from build123d import *

# Parameters (mm, degrees)
SKETCH1_R           = 20.05
SKETCH1_R_2         = 8
BOSS_EXTRUDE1_DEPTH = 8
SKETCH2_R           = 20.05
SKETCH2_R_2         = 8
SKETCH2_R_3         = 20
BOSS_EXTRUDE2_DEPTH = 7
BOSS_EXTRUDE3_START = -2
SKETCH3_R           = 8
SKETCH3_R_2         = 6
BOSS_EXTRUDE3_DEPTH = 2
SKETCH4_R           = 2.5
SKETCH4_R_2         = 1.5
CUT_EXTRUDE1_DEPTH  = 33.0781078
SKETCH5_R           = 2.5
CUT_EXTRUDE2_DEPTH  = 8
CIRPATTERN1_COUNT   = 3
FILLET1_R           = 2
BOSS_EXTRUDE4_START = -1
SKETCH6_R           = 22
SKETCH6_R_2         = 20.05
BOSS_EXTRUDE4_DEPTH = 1
SKETCH7_R           = 2.5
CUT_EXTRUDE3_DEPTH  = 33.124756808


with BuildPart() as part:
    # Sketch1 → Boss-Extrude1 (new body)
    with BuildSketch(Plane(origin=(0, 0, 0), x_dir=(1, 0, 0), z_dir=(0, 1, 0))):
        with Locations(Location((0, 0, 0), (0, 0, 270))):
            Circle(SKETCH1_R)
        with Locations(Location((0, 0, 0), (0, 0, 270))):
            Circle(SKETCH1_R_2, mode=Mode.SUBTRACT)
    extrude(amount=BOSS_EXTRUDE1_DEPTH)

    # Sketch2 → Boss-Extrude2 (add)
    # profile 1 of 2: a face of its own
    with BuildSketch(Plane(origin=(0, 8, 0), x_dir=(1, 0, 0), z_dir=(0, 1, 0))):
        with Locations(Location((0, 0, 0), (0, 0, 270))):
            Circle(SKETCH2_R)
        with Locations(Location((0, 0, 0), (0, 0, 270))):
            Circle(SKETCH2_R_2, mode=Mode.SUBTRACT)
    # profile 2 of 2: a face of its own
    with BuildSketch(Plane(origin=(0, 8, 0), x_dir=(1, 0, 0), z_dir=(0, 1, 0))):
        with Locations(Location((0, 0, 0), (0, 0, 270))):
            Circle(SKETCH2_R)
        Circle(SKETCH2_R_3, mode=Mode.SUBTRACT)
    extrude(amount=BOSS_EXTRUDE2_DEPTH)

    # Sketch3 → Boss-Extrude3 (add)
    with BuildSketch(Plane(origin=(0, 15, 0), x_dir=(1, 0, 0), z_dir=(0, 1, 0)).offset(BOSS_EXTRUDE3_START)):
        with Locations(Location((0, 0, 0), (0, 0, 270))):
            Circle(SKETCH3_R)
        with Locations(Location((0, 0, 0), (0, 0, 270))):
            Circle(SKETCH3_R_2, mode=Mode.SUBTRACT)
    extrude(amount=BOSS_EXTRUDE3_DEPTH)

    # Sketch4 → Cut-Extrude1 (cut, through all)
    with BuildSketch(Plane(origin=(0, 15, 0), x_dir=(1, 0, 0), z_dir=(0, 1, 0))):
        with Locations(Location((0, 16.5, 0), (0, 0, 270))):
            Circle(SKETCH4_R)
        with Locations(Location((14.289419162, -8.25, 0), (0, 0, 270))):
            Circle(SKETCH4_R)
        with Locations(Location((-14.289419162, -8.25, 0), (0, 0, 270))):
            Circle(SKETCH4_R)
        with Locations(Location((0, -16.5, 0), (0, 0, 270))):
            Circle(SKETCH4_R_2)
        with Locations(Location((-14.289419162, 8.25, 0), (0, 0, 270))):
            Circle(SKETCH4_R_2)
        with Locations(Location((14.289419162, 8.25, 0), (0, 0, 270))):
            Circle(SKETCH4_R_2)
    extrude(amount=-CUT_EXTRUDE1_DEPTH, mode=Mode.SUBTRACT)

    # Sketch5 → Cut-Extrude2 (cut)
    with BuildSketch(Plane.XZ):
        with BuildLine():
            ThreePointArc((-3.332922817, 7.272662889), (-2.919714264, 7.448172166), (-2.497311128, 7.600226124))
            Line((-2.497311128, 7.600226124), (-6.258886015, 19.048066722))
            ThreePointArc((-6.258886015, 19.048066722), (-7.661105353, 18.52862555), (-9.020711712, 17.906123539))
            ThreePointArc((-9.020711712, 17.906123539), (-17.363809346, 10.025), (-20.017513724, -1.140896267))
            ThreePointArc((-20.017513724, -1.140896267), (-19.8768131, -2.629600918), (-19.625552682, -4.103679072))
            Line((-19.625552682, -4.103679072), (-7.830644462, -1.637378184))
            ThreePointArc((-7.830644462, -1.637378184), (-7.91016344, -1.195539359), (-7.964772223, -0.749935616))
            ThreePointArc((-7.964772223, -0.749935616), (-6.92820323, 4), (-3.332922817, 7.272662889))
        make_face()
        with Locations(Location((-14.289419162, 8.25, 0), (0, 0, 90))):
            Circle(SKETCH5_R, mode=Mode.SUBTRACT)
    cut_extrude2 = extrude(amount=-CUT_EXTRUDE2_DEPTH, mode=Mode.SUBTRACT)

    # CirPattern1: Cut-Extrude2 ×3 about axis
    cirpattern1_axis = Axis((0, 0, 0), (0, 1, 0))
    for i in range(1, CIRPATTERN1_COUNT):
        add(cut_extrude2.rotate(cirpattern1_axis, i * 360 / CIRPATTERN1_COUNT), mode=Mode.SUBTRACT)

    # Fillet1
    fillet1_edges = [part.edges().sort_by_distance(p)[0] for p in [
        (-7.830644462, 4, -1.637378184),
        (-19.625552682, 4, -4.103679072),
        (-6.258886015, 4, 19.048066722),
        (-2.497311128, 4, 7.600226124),
        (2.497311128, 4, 7.600226124),
        (6.258886015, 4, 19.048066722),
        (19.625552682, 4, -4.103679072),
        (7.830644462, 4, -1.637378184),
        (5.333333333, 4, -5.96284794),
        (13.366666667, 4, -14.94438765),
        (-13.366666667, 4, -14.94438765),
        (-5.333333333, 4, -5.96284794),
    ]]
    fillet(fillet1_edges, radius=FILLET1_R)

    # Sketch6 → Boss-Extrude4 (add)
    with BuildSketch(Plane(origin=(0, 15, 0), x_dir=(1, 0, 0), z_dir=(0, 1, 0)).offset(BOSS_EXTRUDE4_START)):
        with Locations(Location((0, 0, 0), (0, 0, 270))):
            Circle(SKETCH6_R)
        with Locations(Location((0, 0, 0), (0, 0, 41.828059361))):
            Circle(SKETCH6_R_2, mode=Mode.SUBTRACT)
    extrude(amount=BOSS_EXTRUDE4_DEPTH)

    # Sketch7 → Cut-Extrude3 (cut, through all)
    # profile 1 of 2: a face of its own
    with BuildSketch(Plane.XZ.offset(-8)):
        with BuildLine():
            ThreePointArc((4.109756896, 19.624280834), (5.43201172, 18.666478367), (5.599862615, 17.042418804))
            Line((5.599862615, 17.042418804), (3.058568997, 9.308337966))
            ThreePointArc((3.058568997, 9.308337966), (2.235430366, 8.247362264), (0.926809973, 7.946132599))
            ThreePointArc((0.926809973, 7.946132599), (6.92820323, 4), (7.344957679, -3.170425319))
            ThreePointArc((7.344957679, -3.170425319), (8.260140418, -2.187741646), (9.590541644, -2.005370533))
            Line((9.590541644, -2.005370533), (17.559098934, -3.67158612))
            ThreePointArc((17.559098934, -3.67158612), (18.881650325, -4.62897904), (19.050004181, -6.252986541))
            ThreePointArc((19.050004181, -6.252986541), (17.363809346, 10.025), (4.109756896, 19.624280834))
        make_face()
        with Locations(Location((14.289419162, 8.25, 0), (0, 0, 90))):
            Circle(SKETCH7_R, mode=Mode.SUBTRACT)
    # profile 2 of 2: a face of its own
    with BuildSketch(Plane.XZ.offset(-8)):
        with BuildLine():
            ThreePointArc((5.599862615, 17.042418804), (5.43201172, 18.666478367), (4.109756896, 19.624280834))
            ThreePointArc((4.109756896, 19.624280834), (-17.363809346, -10.025), (19.050004181, -6.252986541))
            ThreePointArc((19.050004181, -6.252986541), (18.881650325, -4.62897904), (17.559098934, -3.67158612))
            Line((17.559098934, -3.67158612), (9.590541644, -2.005370533))
            ThreePointArc((9.590541644, -2.005370533), (8.260140418, -2.187741646), (7.344957679, -3.170425319))
            ThreePointArc((7.344957679, -3.170425319), (-6.92820323, -4), (0.926809973, 7.946132599))
            ThreePointArc((0.926809973, 7.946132599), (2.235430366, 8.247362264), (3.058568997, 9.308337966))
            Line((3.058568997, 9.308337966), (5.599862615, 17.042418804))
        make_face()
    extrude(amount=CUT_EXTRUDE3_DEPTH, mode=Mode.SUBTRACT)


solid = part.part
Build history of the part. All positions in model axes, mm. A direction names the side the tool comes from. Coordinates: 2 decimals unless noted, no trailing zeros. Order: outer loops, then holes, each group sorted by start corner. A loop starts at its lowest first (then second) coordinate and runs counter-clockwise, first axis right, second up. Notation, with made-up numbers: (36, 49) -> (61, 49) arc R16 cw to (61, 58) -> close; hole circle Ø6 at (27.5, 70.5). An arc over 180 degrees is marked (long way). One line per item, written item: value.
(1) Mould opens along Z. For faces 1 (the flat face through (-5, 15, 5)), 2 (the cylindrical face through (6.022, 10.958, 19.124)), 3 (the cylindrical face through (15.777, 11.549, -8.445)) say: pulls with the +Z half, pulls with the -Z half, needs draft (parallel to the pull), parting line crosses it, or undercut.
Checked values:
face 1: needs draft
face 2: parting line crosses it
face 3: undercut
(2) Slice it at B-B, the plane z = 0. List the corners of the cut face in (x, y), plus the area to 3 significant figures.
Checked values:
outline: (-22, 14) -> (-20.05, 14) -> (-20.05, 8) -> (-8, 8) -> (-8, 13) -> (-6, 13) -> (-6, 15) -> (-22, 15) -> close; (6, 13) -> (8, 13) -> (8, 8) -> (20.05, 8) -> (20.05, 14) -> (22, 14) -> (22, 15) -> (6, 15) -> close
area: 181 mm2
(3) Slice it at C-C, the plane y = 9.5. List the corners of the cut face in (x, z), plus the area to 3 significant figures.
Checked values:
outline: circle Ø40.1 at (0, 0); hole circle Ø5 at (-14.29, 8.25); hole circle Ø3 at (-14.29, -8.25); hole circle Ø16 at (0, 0); hole circle Ø5 at (0, -16.5); hole circle Ø3 at (0, 16.5); hole circle Ø5 at (14.29, 8.25); hole circle Ø3 at (14.29, -8.25)
area: 982 mm2
(4) Probe line 1 (X direction, y = 14.5, z = 0); line 2 (X direction, y = 10.5, z = 8.25); line 3 (X direction, y = 10, z = -8.25). List the from-to ranges inside material, lowest first. Write a range as [from, to].
Checked values:
line 1: [-22, -6], [6, 22]
line 2: [-18.27, -16.79], [-11.79, 11.79], [16.79, 18.27]
line 3: [-18.27, -15.79], [-12.79, 12.79], [15.79, 18.27]
(5) Tool access for faces 4 (the flat face through (-10, 14, 18)), 5 (the cylindrical face through (0, 12, 15)): list every direction of +Z, -Z, +X, -X, +Y, -Y with a clear straight run to the whole face (end or side of a thin tool).
Checked values:
face 4: -Y
face 5: +Y, -Y
(6) Slice it at D-D, the plane z = 16.5. List the corners of the cut face in (x, y), plus the area to 3 significant figures.
Checked values:
outline: (-14.55, 14) -> (-11.39, 14) -> (-11.39, 8) -> (-1.5, 8) -> (-1.5, 15) -> (-14.55, 15) -> close; (1.5, 8) -> (11.39, 8) -> (11.39, 14) -> (14.55, 14) -> (14.55, 15) -> (1.5, 15) -> close
area: 145 mm2
(7) Slice it at A-A, the plane x = 0. List the corners of the cut face in (y, z).
Checked values:
outline: (8, -20.05) -> (14, -20.05) -> (14, -22) -> (15, -22) -> (15, -19) -> (8, -19) -> close; (8, -14) -> (15, -14) -> (15, -6) -> (13, -6) -> (13, -8) -> (8, -8) -> close; (8, 8) -> (13, 8) -> (13, 6) -> (15, 6) -> (15, 15) -> (8, 15) -> close; (8, 18) -> (15, 18) -> (15, 22) -> (14, 22) -> (14, 20.05) -> (8, 20.05) -> close
(8) Drop flat-ended pins along their axis: pin 1 Ø7 at (x, z) = (0, 0) entering from -Y; pin 2 Ø1.5 at (y, z) = (11, 3.5) entering from +X; pin 3 Ø4 at (x, y) = (3.5, 8.5) entering from +Z; pin 4 Ø3 at (y, z) = (11.5, -12.5) entering from +X. Give the stop position or say it passes through.
Checked values:
pin 1: through
pin 2: x = 19.86
pin 3: z = 19.99
pin 4: x = 16.76
